The listing builds one solid part. Answer for the finished solid, in the listing's coordinates (mm). A direction names the side the tool comes from. Give positions to 0.01 mm unless a question says otherwise; leave off trailing zeros. Order: outer loops, then holes, each group sorted by start corner. A loop starts at its lowest first (then second) coordinate and runs counter-clockwise, first axis right, second up. Notation, with made-up numbers: (-13.5, -21.75) - (0.5, -21.75) arc R5 cw to (0.5, -17.75) - close; hole circle Ø9 at (42.5, 0.25). An arc over 180 degrees is marked (long way). Use a Markdown table: item, result. Add a question column.
1) Flat-ended cylindrical pins translate along their axes: pin 1 (1.2 mm diameter, centred on x = -25, y = 29, fed in from +Z); pin 2 (3 mm diameter, centred on x = -25.5, y = 28.79, fed in from -Z); pin 3 (6 mm diameter, centred on x = -14.5, z = -9, fed in from +Y); pin 4 (5 mm diameter, centred on x = 24.5, z = -10.5, fed in from +Y). Find the tip coordinate at first contact, or state that the pin passes through.
2) Find section C-C, the plane y = 8.5. Determine the outline of the cut face in (x, z) (3 decimals).
3) Find section B-B, the plane z = 1.5. Determine the outline of the cut face in (x, y) (3 decimals), plus the area to 3 significant figures.
4) Straight lines are drawn through the part: line 1 (Y direction, x = 25.5, z = 15.2); line 2 (X direction, y = 19, z = 15) (3 decimals); line 3 (X direction, y = 31, z = 15) (3 decimals). For each, find the intervals that lie inside material, in ascending order.
5) Find section D-D, the plane y = 19.05. State how many separate pieces and enclosed holes the cut face has, plus the area to 3 significant figures.
6) The mould has two halves that part along X. Classify faces 1 (the face through (23.9, 27.56, 16.36)), 2 (the face through (-20.481, 0, -2)), 3 (the face through (29, 18, 19.05)): released by +X, released by -X, zero draft, split by the parting line, or undercut.
7) Find section A-A, the plane z = -25. Determine the outline of the cut face in (x, y) (1 decimal), plus the area to 3 significant figures.
8) For faces 4 (the face through (-26, 29, 13.589)), 5 (the face through (17, -2.54, -21)), 6 (the face through (-2.54, -17, -21)), determine the directions among +Z, -Z, +X, -X, +Y, -Y from which every point of the face is accessible in a straight line to the end or side of a thin tool.
from build123d import *

# Parameters (mm, degrees)
BOSS_EXTRUDE3_DEPTH   = 31.75
BOSS_EXTRUDE3_2_DEPTH = 31.75
BOSS_EXTRUDE3_3_DEPTH = 31.75
BOSS_EXTRUDE3_4_DEPTH = 31.75
BOSS_EXTRUDE4_DEPTH   = 5.08
CIRPATTERN2_COUNT     = 4
CUT_EXTRUDE1_DEPTH    = 47.752
BOSS_EXTRUDE6_DEPTH   = 19.05
SKETCH12_R            = 2.0193
CUT_EXTRUDE2_DEPTH    = 5.461
FILLET5_R             = 2.54


with BuildPart() as part:
    # Sketch4 → Boss-Extrude3 (new body)
    with BuildSketch(Plane.XY):
        with BuildLine():
            Line((-20.480595847, 2.54), (-12.443407893, 2.54))
            ThreePointArc((-12.443407893, 2.54), (-8.980256121, 8.980256121), (-2.54, 12.443407893))
            Line((-2.54, 12.443407893), (-2.54, 20.480595847))
            ThreePointArc((-2.54, 20.480595847), (-14.592916197, 14.592916197), (-20.480595847, 2.54))
        make_face()
    extrude(amount=-BOSS_EXTRUDE3_DEPTH)


with BuildPart() as body_2:
    # Sketch4 → Boss-Extrude3 2 (new body)
    with BuildSketch(Plane.XY):
        with BuildLine():
            ThreePointArc((-2.54, -12.443407893), (-8.980256121, -8.980256121), (-12.443407893, -2.54))
            Line((-12.443407893, -2.54), (-20.480595847, -2.54))
            ThreePointArc((-20.480595847, -2.54), (-14.592916197, -14.592916197), (-2.54, -20.480595847))
            Line((-2.54, -20.480595847), (-2.54, -12.443407893))
        make_face()
    extrude(amount=-BOSS_EXTRUDE3_2_DEPTH)


with BuildPart() as body_3:
    # Sketch4 → Boss-Extrude3 3 (new body)
    with BuildSketch(Plane.XY):
        with BuildLine():
            Line((2.54, 20.480595847), (2.54, 12.443407893))
            ThreePointArc((2.54, 12.443407893), (8.980256121, 8.980256121), (12.443407893, 2.54))
            Line((12.443407893, 2.54), (20.480595847, 2.54))
            ThreePointArc((20.480595847, 2.54), (14.592916197, 14.592916197), (2.54, 20.480595847))
        make_face()
    extrude(amount=-BOSS_EXTRUDE3_3_DEPTH)


with BuildPart() as body_4:
    # Sketch4 → Boss-Extrude3 4 (new body)
    with BuildSketch(Plane.XY):
        with BuildLine():
            ThreePointArc((12.443407893, -2.54), (8.980256121, -8.980256121), (2.54, -12.443407893))
            Line((2.54, -12.443407893), (2.54, -20.480595847))
            ThreePointArc((2.54, -20.480595847), (14.592916197, -14.592916197), (20.480595847, -2.54))
            Line((20.480595847, -2.54), (12.443407893, -2.54))
        make_face()
    extrude(amount=-BOSS_EXTRUDE3_4_DEPTH)


with BuildPart() as body_5:
    # Sketch7 → Boss-Extrude4 (new body)
    with BuildSketch(Plane.XZ.offset(-2.54)):
        Polygon((12.443407893, 0), (12.443407893, -11.847187954), (20.480595847, -3.81), (20.480595847, 0), align=None)
    extrude(amount=BOSS_EXTRUDE4_DEPTH)


with BuildPart() as cirpattern2_1:
    # CirPattern2: pattern copy
    add(body_5.part.rotate(Axis((0, 0, 0), (0, 0, 1)), 1 * 360 / CIRPATTERN2_COUNT))


with BuildPart() as cirpattern2_2:
    # CirPattern2: pattern copy
    add(body_5.part.rotate(Axis((0, 0, 0), (0, 0, 1)), 2 * 360 / CIRPATTERN2_COUNT))


with BuildPart() as cirpattern2_3:
    # CirPattern2: pattern copy
    add(body_5.part.rotate(Axis((0, 0, 0), (0, 0, 1)), 3 * 360 / CIRPATTERN2_COUNT))


with BuildPart() as body_3_1:
    add(body_3.part)

    # Combine1: union CirPattern2_2, body 2, CirPattern2_3, body 4, body 5, CirPattern2_1, part
    add(cirpattern2_2.part)
    add(body_2.part)
    add(cirpattern2_3.part)
    add(body_4.part)
    add(body_5.part)
    add(cirpattern2_1.part)
    add(part.part)

    # Sketch8 → Cut-Extrude1 (cut)
    with BuildSketch(Plane.XY):
        with BuildLine():
            Line((-2.54, 12.443407893), (2.54, 12.443407893))
            ThreePointArc((2.54, 12.443407893), (0, 12.7), (-2.54, 12.443407893))
        make_face()
        with BuildLine():
            Line((12.443407893, 2.54), (12.443407893, -2.54))
            ThreePointArc((12.443407893, -2.54), (12.635689143, -1.276463817), (12.7, 0))
            ThreePointArc((12.7, 0), (12.635689143, 1.276463817), (12.443407893, 2.54))
        make_face()
        with BuildLine():
            ThreePointArc((-2.54, -12.443407893), (0, -12.7), (2.54, -12.443407893))
            Line((2.54, -12.443407893), (-2.54, -12.443407893))
        make_face()
        with BuildLine():
            ThreePointArc((-12.443407893, 2.54), (-12.7, 0), (-12.443407893, -2.54))
            Line((-12.443407893, -2.54), (-12.443407893, 2.54))
        make_face()
    extrude(amount=-CUT_EXTRUDE1_DEPTH, mode=Mode.SUBTRACT)

    # Sketch11 → Boss-Extrude6 (add)
    with BuildSketch(Plane.XY):
        Polygon((-19.785000054, 33.446844079), (-32.485000054, 33.446844079), (-32.485000054, 14.396844079), (-32.485000054, 2.966844079), (-19.785000054, 2.966844079), align=None)
        Polygon((32.485000054, 33.446844079), (32.485000054, 14.396844079), (32.485000054, 2.966844079), (19.785000054, 2.966844079), (19.785000054, 33.446844079), align=None)
    extrude(amount=BOSS_EXTRUDE6_DEPTH)

    # Sketch12 → Cut-Extrude2 (cut)
    with BuildSketch(Plane.XY.offset(19.05)):
        with Locations((25.500000054, 28.793688158)):
            Circle(SKETCH12_R)
        with Locations((25.500000054, 19.05)):
            Circle(SKETCH12_R)
        with Locations((-25.500000054, 28.793688158)):
            Circle(SKETCH12_R)
        with Locations((-25.500000054, 19.05)):
            Circle(SKETCH12_R)
    extrude(amount=-CUT_EXTRUDE2_DEPTH, mode=Mode.SUBTRACT)

    # Fillet5
    fillet5_edges = [body_3_1.edges().sort_by_distance(p)[0] for p in [
        (-19.785000054, 18.206844079, 19.05),
        (19.785000054, 18.206844079, 19.05),
    ]]
    fillet(fillet5_edges, radius=FILLET5_R)


solid = body_3_1.part
The answers:
| question | item | result |
|---|---|---|
| 1 | pin 1 | z = 13.59 |
| 1 | pin 2 | z = 0 |
| 1 | pin 3 | y = 17.14 |
| 1 | pin 4 | through |
| 2 | outline | (-32.485, 0) - (-19.785, 0) - (-19.785, 16.51) arc R2.54 ccw to (-22.325, 19.05) - (-32.485, 19.05) - close; (-18.806, -31.75) - (-9.436, -31.75) - (-9.436, 0) - (-18.806, 0) - close; (9.436, -31.75) - (18.806, -31.75) - (18.806, 0) - (9.436, 0) - close; (19.785, 0) - (32.485, 0) - (32.485, 19.05) - (22.325, 19.05) arc R2.54 ccw to (19.785, 16.51) - close |
| 3 | outline | (-32.485, 2.967) - (-19.785, 2.967) - (-19.785, 33.447) - (-32.485, 33.447) - close; (19.785, 2.967) - (32.485, 2.967) - (32.485, 33.447) - (19.785, 33.447) - close |
| 3 | area | 774 mm2 |
| 4 | line 1 | 2.97 to 17.03, 21.07 to 26.77, 30.81 to 33.45 |
| 4 | line 2 | -32.485 to -27.519, -23.481 to -19.785, 19.785 to 23.481, 27.519 to 32.485 |
| 4 | line 3 | -32.485 to -19.785, 19.785 to 32.485 |
| 5 | separate pieces | 3 |
| 5 | enclosed holes | 0 |
| 5 | area | 806 mm2 |
| 6 | face 1 | undercut |
| 6 | face 2 | released by -X |
| 6 | face 3 | zero draft |
| 7 | outline | (-20.5, -2.5) arc R20.6 ccw to (-2.5, -20.5) - (-2.5, -12.4) arc R12.7 cw to (-12.4, -2.5) - close; (-20.5, 2.5) - (-12.4, 2.5) arc R12.7 cw to (-2.5, 12.4) - (-2.5, 20.5) arc R20.6 ccw to start; (2.5, -20.5) arc R20.6 ccw to (20.5, -2.5) - (12.4, -2.5) arc R12.7 cw to (2.5, -12.4) - close; (2.5, 12.4) arc R12.7 cw to (12.4, 2.5) - (20.5, 2.5) arc R20.6 ccw to (2.5, 20.5) - close |
| 7 | area | 669 mm2 |
| 8 | face 4 | +Z |
| 8 | face 5 | -Z, +X |
| 8 | face 6 | -Z, -Y |
